Read the model definition and answer for the solid it produces. Units are mm, in the model's axes. A direction names the side the tool comes from. Coordinates: 2 decimals unless noted, no trailing zeros. Write each loop counter-clockwise with the first axis right and the second up, starting at its lowest first coordinate (ties: lowest second). Pieces come first, ordered by that corner, then holes. Notation, with made-up numbers: M 76,-22 L 112,-22 A27 cw 112,1 Z; hole C 79.5,78.5 d11. An arc over 180 degrees is marked long. Write item = value, one per line.
from build123d import *

# Parameters (mm, degrees)
SKIZZE1_W                                            = 110
SKIZZE1_H                                            = 100
AUFSATZ_LINEAR_AUSTRAGEN1_DEPTH                      = 25
VERRUNDUNG1_R                                        = 5
STIRNSENKUNG_F_R_M12_ZYLINDERSCHRAUBE_MI_D           = 13.5
STIRNSENKUNG_F_R_M12_ZYLINDERSCHRAUBE_MI_CBORE_D     = 20
STIRNSENKUNG_F_R_M12_ZYLINDERSCHRAUBE_MI_CBORE_DEPTH = 8.1
F_10_0MM_STIFTLOCH1_D                                = 10
F_10_0MM_STIFTLOCH1_DEPTH                            = 10
F_10_0MM_STIFTLOCH1_TIP                              = 3.004303095


with BuildPart() as part:
    # Skizze1 → Aufsatz-Linear austragen1 (new body)
    with BuildSketch(Plane.XY):
        Rectangle(SKIZZE1_W, SKIZZE1_H)
    extrude(amount=AUFSATZ_LINEAR_AUSTRAGEN1_DEPTH)

    # Verrundung1
    verrundung1_edges = [part.edges().sort_by_distance(p)[0] for p in [
        (55, -50, 12.5),
        (-55, -50, 12.5),
        (-55, 50, 12.5),
        (55, 50, 12.5),
    ]]
    fillet(verrundung1_edges, radius=VERRUNDUNG1_R)

    # Stirnsenkung für M12 Zylinderschraube mit Innensechskant1 (through all)
    with Locations(Plane.XY.offset(25)):
        with Locations((-41, 27.5), (41, 27.5), (41, -27.5), (-41, -27.5)):
            CounterBoreHole(STIRNSENKUNG_F_R_M12_ZYLINDERSCHRAUBE_MI_D / 2, STIRNSENKUNG_F_R_M12_ZYLINDERSCHRAUBE_MI_CBORE_D / 2, STIRNSENKUNG_F_R_M12_ZYLINDERSCHRAUBE_MI_CBORE_DEPTH)

    # Ø10.0mm Stiftloch1
    with Locations(Plane.XY.offset(25)):
        with Locations((0, 20), (0, -20)):
            Hole(F_10_0MM_STIFTLOCH1_D / 2, depth=F_10_0MM_STIFTLOCH1_DEPTH)
            with Locations((0, 0, -(F_10_0MM_STIFTLOCH1_DEPTH + F_10_0MM_STIFTLOCH1_TIP / 2))):  # 118° drill point
                Cone(0, F_10_0MM_STIFTLOCH1_D / 2, F_10_0MM_STIFTLOCH1_TIP, mode=Mode.SUBTRACT)


solid = part.part
Item 1: Which of the six approach directions +Z, -Z, +X, -X, +Y, -Y give full straight-line access (tool end or side, diameter ignored) to faces 1 (the face through (-1, 1, 0)), 2 (the face through (-34, 25, 16.9))?
Worked answers:
face_1 = -Z, +X, -X, +Y, -Y
face_2 = +Z
Item 2: Flat-ended cylindrical pins translate along their axes: pin 1 (10 mm diameter, centred on x = -43.5, y = 29, fed in from +Z); pin 2 (6 mm diameter, centred on x = 0, y = -20, fed in from +Z). Find the tip coordinate at first contact, or state that the pin passes through.
Worked answers:
pin_1 = 16.9
pin_2 = 13.8
Item 3: Find section C-C (z = 19.5). Determine the outline of the cut face in (x, y), and give its area (3 significant figures).
Worked answers:
outline = M -55,-45 A5 ccw -50,-50 L 50,-50 A5 ccw 55,-45 L 55,45 A5 ccw 50,50 L -50,50 A5 ccw -55,45 Z; hole C -41,-27.5 d20; hole C -41,27.5 d20; hole C 0,-20 d10; hole C 0,20 d10; hole C 41,-27.5 d20; hole C 41,27.5 d20
area = 9,560 mm²
Item 4: Find section D-D (y = -30.5). Determine the outline of the cut face in (x, z).
Worked answers:
outline = M -55,0 L -47.05,0 L -47.05,16.9 L -50.54,16.9 L -50.54,25 L -55,25 Z; M -34.95,0 L 34.95,0 L 34.95,16.9 L 31.46,16.9 L 31.46,25 L -31.46,25 L -31.46,16.9 L -34.95,16.9 Z; M 47.05,0 L 55,0 L 55,25 L 50.54,25 L 50.54,16.9 L 47.05,16.9 Z
Item 5: Consider line 1 along Y through (x, z) = (41, 10.5); line 2 along Y through (x, z) = (-41, 22); line 3 along X through (y, z) = (31, 18). Determine where each line is inside the solid, lowest interval first. Write a range as from..to.
Worked answers:
line_1 = -50..-34.25, -20.75..20.75, 34.25..50
line_2 = -50..-37.5, -17.5..17.5, 37.5..50
line_3 = -55..-50.37, -31.63..31.63, 50.37..55
Item 6: Find section B-B (z = 7.5). Determine the outline of the cut face in (x, y), and give its area (3 significant figures).
Worked answers:
outline = M -55,-45 A5 ccw -50,-50 L 50,-50 A5 ccw 55,-45 L 55,45 A5 ccw 50,50 L -50,50 A5 ccw -55,45 Z; hole C -41,-27.5 d13.5; hole C -41,27.5 d13.5; hole C 41,-27.5 d13.5; hole C 41,27.5 d13.5
area = 10,400 mm²
Item 7: For a pull along X with two mould halves and no side action, classify faces 3 (the face through (-54, -48, 13)), 4 (the face through (-1, 50, 12)), 5 (the face through (48, -30, 16.9)) as released by +X, released by -X, zero draft, split by the parting line, or undercut.
Worked answers:
face_3 = released by -X
face_4 = zero draft
face_5 = undercut
Item 8: Find section A-A (x = 41). Determine the outline of the cut face in (y, z), and give its area (3 significant figures).
Worked answers:
outline = M -50,0 L -34.25,0 L -34.25,16.9 L -37.5,16.9 L -37.5,25 L -50,25 Z; M -20.75,0 L 20.75,0 L 20.75,16.9 L 17.5,16.9 L 17.5,25 L -17.5,25 L -17.5,16.9 L -20.75,16.9 Z; M 34.25,0 L 50,0 L 50,25 L 37.5,25 L 37.5,16.9 L 34.25,16.9 Z
area = 1,720 mm²
